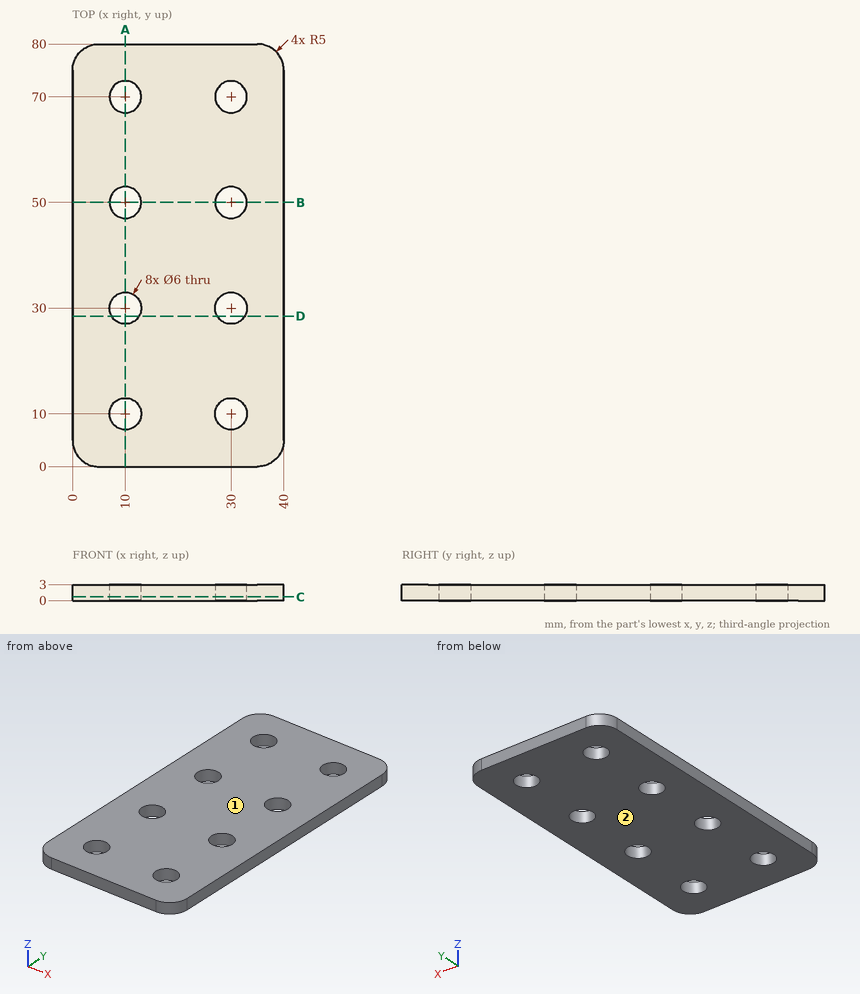
Check sheet for the drawn part. Datum: minimum x, y, z corner. Units: mm. Coordinates: 2 decimals unless noted, no trailing zeros. Order: outer loops, then holes, each group sorted by start corner. A loop starts at its lowest first (then second) coordinate and runs counter-clockwise, first axis right, second up. Notation, with made-up numbers: (-35.5, 0) -> (-3.5, 0) arc R15 ccw to (-3.5, 29) -> close; hole circle Ø3 at (85.5, 75.5). An arc over 180 degrees is marked (long way). Write each question's results on one line, items separated by ' | '. Start each with the question number.
1) Section check C-C (z = 0.7). Count the separate pieces of the cut face and the enclosed holes in it, and give its area (3 significant figures).
2) Material ranges on line 1 along Y through (x, z) = (10, 0.8); line 2 along X through (y, z) = (30, 2); line 3 along Y through (x, z) = (12.5, 1.7), recorded low to high.
3) Section check B-B (y = 50). Enter the section's corners in (x, z).
4) Section check D-D (y = 28.5). Enter the section's corners in (x, z).
5) Draft check along Z on the marked faces 1 and 2. Enter one of: pulls with the +Z half, pulls with the -Z half, needs draft (parallel to the pull), parting line crosses it, or undercut.
6) Section check A-A (x = 10). Enter the section's corners in (y, z).
Checked values:
1) separate pieces: 1 | enclosed holes: 8 | area: 2,950 mm²
2) line 1: 0 to 7, 13 to 27, 33 to 47, 53 to 67, 73 to 80 | line 2: 0 to 7, 13 to 27, 33 to 40 | line 3: 0 to 8.34, 11.66 to 28.34, 31.66 to 48.34, 51.66 to 68.34, 71.66 to 80
3) outline: (0, 0) -> (7, 0) -> (7, 3) -> (0, 3) -> close; (13, 0) -> (27, 0) -> (27, 3) -> (13, 3) -> close; (33, 0) -> (40, 0) -> (40, 3) -> (33, 3) -> close
4) outline: (0, 0) -> (7.4, 0) -> (7.4, 3) -> (0, 3) -> close; (12.6, 0) -> (27.4, 0) -> (27.4, 3) -> (12.6, 3) -> close; (32.6, 0) -> (40, 0) -> (40, 3) -> (32.6, 3) -> close
5) face 1: pulls with the +Z half | face 2: pulls with the -Z half
6) outline: (0, 0) -> (7, 0) -> (7, 3) -> (0, 3) -> close; (13, 0) -> (27, 0) -> (27, 3) -> (13, 3) -> close; (33, 0) -> (47, 0) -> (47, 3) -> (33, 3) -> close; (53, 0) -> (67, 0) -> (67, 3) -> (53, 3) -> close; (73, 0) -> (80, 0) -> (80, 3) -> (73, 3) -> close
